The listing builds one solid part. Answer for the finished solid, in the listing's coordinates (mm). Face numbers are marked on the shaded views. Give positions to 0.01 mm unless a question says otherwise; leave off trailing zeros. Write each loop counter-clockwise with the first axis right and the second up, starting at its lowest first coordinate (ties: lowest second). Pieces come first, ordered by that corner, then holes.
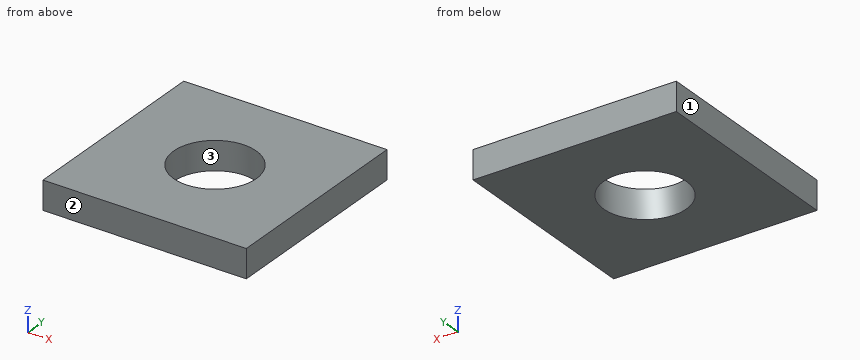
Autodesk Inventor part; units mm, degrees
ref_plane "YZ Plane" through (0, 0, 0) normal (1, 0, 0) x (0, 1, 0)
ref_plane "XZ Plane" through (0, 0, 0) normal (0, 1, 0) x (-1, 0, 0)
ref_plane "XY Plane" through (0, 0, 0) normal (0, 0, 1) x (1, 0, 0)
sketch "スケッチ1" plane through (0, 0, 0) normal (0, 0, 1) x (1, 0, 0)
  line L0 (-16, -16) -> (16, -16)
  line L1 (16, -16) -> (16, 16)
  line L2 (16, 16) -> (-16, 16)
  line L3 (-16, 16) -> (-16, -16)
  line L4 (-16, -16) -> (16, 16) construction
  line L5 (16, -16) -> (-16, 16) construction
  point P0 (0, 0)
  dimension "d0" = 32
  dimension "d1" = 32
extrude "押し出し1" add sketch "スケッチ1" along normal blind 4.5
sketch "スケッチ2" plane through (0, 0, 4.5) normal (0, 0, 1) x (1, 0, 0)
  point P0 (0, 0)
  point P1 (0, 0)
hole "穴1" at (0, 0, 4.5) direction (0, 0, -1) diameter 13 end through all
properties part number "PipeB蓋"
Item 1: A cutting plane is placed at A-A, the plane x = 0. Give the vertices of the cut face in (y, z), plus the area to 3 significant figures.
Conclusion:
outline: (-16, 0) - (-6.5, 0) - (-6.5, 4.5) - (-16, 4.5) - close; (6.5, 0) - (16, 0) - (16, 4.5) - (6.5, 4.5) - close
area: 85.5 mm2
Item 2: A cutting plane is placed at C-C, the plane z = 0.6. Give the vertices of the cut face in (x, y).
Conclusion:
outline: (-16, -16) - (16, -16) - (16, 16) - (-16, 16) - close; hole circle Ø13 at (0, 0)
Item 3: Consider probe 1 along X at (y, z) = (0, 1.95); probe 2 along Y at (x, z) = (-5.5, 1.8). Determine where each line is inside the solid, lowest interval first.
Conclusion:
probe 1: x = -16 to -6.5, 6.5 to 16
probe 2: y = -16 to -3.46, 3.46 to 16
Item 4: Determine the mould class of the marked faces 1, 2 and 3 for opening direction X: pulls with the +X half, pulls with the -X half, needs draft (parallel to the pull), parting line crosses it, or undercut.
Conclusion:
face 1: pulls with the -X half
face 2: needs draft
face 3: undercut
